Input: part model. Units: mm. Frame: model coordinates. A direction names the side the tool comes from. Round coordinates to 2 decimals unless told otherwise and drop trailing zeros. Loops run counter-clockwise (first coordinate to the right, second up) from the corner with the lowest first, then second, coordinate; pieces in that order, holes last. Notation, with made-up numbers: (34.5, 81) -> (70.5, 81) arc R12 ccw to (70.5, 87) -> close; hole circle Ø11 at (44.25, 84). An arc over 180 degrees is marked (long way). Answer as a JSON object with one key per item and string values.
```python
from build123d import *

# Parameters (mm, degrees)
SKETCH_1_W          = 100
SKETCH_1_H          = 100
EXTRUDE_3_DEPTH     = 8
SKETCH_4_W          = 100
SKETCH_4_H          = 100
SKETCH_4_W_2        = 94
SKETCH_4_H_2        = 94
SKETCH_4_W_3        = 88
SKETCH_4_H_3        = 88
CUT_EXTRUDE_3_DEPTH = 5


with BuildPart() as part:
    # 草图1 → 凸台-拉伸3 (new body)
    with BuildSketch(Plane.XY):
        with Locations((1.458885942, 2.519893899)):
            Rectangle(SKETCH_1_W, SKETCH_1_H)
    extrude(amount=EXTRUDE_3_DEPTH)

    # 草图4 → 切除-拉伸3 (cut)
    with BuildSketch(Plane.XY.offset(8)):
        with Locations((1.458885942, 2.519893899)):
            Rectangle(SKETCH_4_W, SKETCH_4_H)
        with Locations((1.458885942, 2.519893899)):
            Rectangle(SKETCH_4_W_2, SKETCH_4_H_2, mode=Mode.SUBTRACT)
        with Locations((1.458885942, 2.519893899)):
            Rectangle(SKETCH_4_W_3, SKETCH_4_H_3)
    extrude(amount=-CUT_EXTRUDE_3_DEPTH, mode=Mode.SUBTRACT)


solid = part.part
```
1) Ray query, probe 1 along Y at (x, z) = (-38.5, 4.5); probe 2 along X at (y, z) = (41, 4.75); probe 3 along Z at (x, y) = (-19.5, 15). Return the intervals inside material, ascending.
Output:
{"probe 1": "y = -44.48 to -41.48, 46.52 to 49.52", "probe 2": "x = -45.54 to -42.54, 45.46 to 48.46", "probe 3": "z = 0 to 3"}
2) Contact query for flat-ended pins moving along their axis: P1, Ø4, axis at y = 20.5, z = 6, coming from the +X side; P2, Ø2, axis at x = 21.5, z = 5, coming from the -Y side; P3, Ø10, axis at x = 14.5, y = -11.5, coming from the +Z side. Output: stop coordinate, or through.
Output:
{"P1": "stops at x = 48.46", "P2": "stops at y = -44.48", "P3": "stops at z = 3"}
3) Section B-B, the plane x = 40.5. Output: boundary loops of the cut face in (y, z), plus the area to 3 significant figures.
Output:
{"outline": "(-47.48, 0) -> (52.52, 0) -> (52.52, 3) -> (49.52, 3) -> (49.52, 8) -> (46.52, 8) -> (46.52, 3) -> (-41.48, 3) -> (-41.48, 8) -> (-44.48, 8) -> (-44.48, 3) -> (-47.48, 3) -> close", "area": "330 mm^2"}
4) Reachability of faces 1 (the face through (1, -44.48, 6)), 2 (the face through (1, 46.52, 6)), 3 (the face through (48.459, 2, 6)) from +Z, -Z, +X, -X, +Y, -Y: full face, straight path, thin tool, end or side. Return the list, or none.
Output:
{"face 1": "+Z, +X, -X, -Y", "face 2": "+Z", "face 3": "+Z, +X, +Y, -Y"}
5) Draft query along X for faces 4 (the face through (-45.541, 2, 6)), 5 (the face through (-2, -43, 8)), 6 (the face through (-42.541, 2, 6)). Return one class per face: +X half, -X half, draft (parallel to the pull), parting line (faces both ways), or undercut.
Output:
{"face 4": "-X half", "face 5": "draft", "face 6": "undercut"}
6) Section C-C, the plane y = 26. Output: boundary loops of the cut face in (x, z), plus the area to 3 significant figures.
Output:
{"outline": "(-48.54, 0) -> (51.46, 0) -> (51.46, 3) -> (48.46, 3) -> (48.46, 8) -> (45.46, 8) -> (45.46, 3) -> (-42.54, 3) -> (-42.54, 8) -> (-45.54, 8) -> (-45.54, 3) -> (-48.54, 3) -> close", "area": "330 mm^2"}
7) Section A-A, the plane z = 6. Output: boundary loops of the cut face in (x, y).
Output:
{"outline": "(-45.54, -44.48) -> (48.46, -44.48) -> (48.46, 49.52) -> (-45.54, 49.52) -> close; hole (-42.54, -41.48) -> (45.46, -41.48) -> (45.46, 46.52) -> (-42.54, 46.52) -> close"}
